from build123d import *

# Parameters (mm, degrees)
CROQUIS1_W              = 70
CROQUIS1_H              = 70
CROQUIS1_R              = 25.5
SALIENTE_EXTRUIR1_DEPTH = 2
CROQUIS2_R              = 27.5
CROQUIS2_R_2            = 25.5
SALIENTE_EXTRUIR2_DEPTH = 3
CROQUIS3_W              = 70
CROQUIS3_H              = 17
CORTAR_EXTRUIR1_DEPTH   = 50.749371855


with BuildPart() as part:
    # Croquis1 → Saliente-Extruir1 (new body)
    with BuildSketch(Plane(origin=(0, 0, 0), x_dir=(1, 0, 0), z_dir=(0, 1, 0))):
        Rectangle(CROQUIS1_W, CROQUIS1_H)
        with Locations(Location((0, 0, 0), (0, 0, 270))):
            Circle(CROQUIS1_R, mode=Mode.SUBTRACT)
    extrude(amount=SALIENTE_EXTRUIR1_DEPTH)

    # Croquis2 → Saliente-Extruir2 (add)
    with BuildSketch(Plane(origin=(0, 2, 0), x_dir=(1, 0, 0), z_dir=(0, 1, 0))):
        with Locations(Location((0, 0, 0), (0, 0, 270))):
            Circle(CROQUIS2_R)
        with Locations(Location((0, 0, 0), (0, 0, 270))):
            Circle(CROQUIS2_R_2, mode=Mode.SUBTRACT)
    extrude(amount=SALIENTE_EXTRUIR2_DEPTH)

    # Croquis3 → Cortar-Extruir1 (cut, through all)
    with BuildSketch(Plane(origin=(0, 5, 0), x_dir=(1, 0, 0), z_dir=(0, 1, 0))):
        with Locations((0, -26.5)):
            Rectangle(CROQUIS3_W, CROQUIS3_H)
    extrude(amount=-CORTAR_EXTRUIR1_DEPTH, mode=Mode.SUBTRACT)


solid = part.part
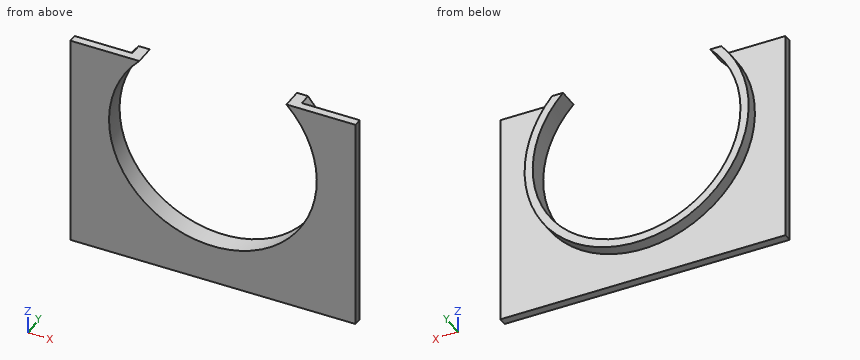
Design review of the part built by this model. Coordinates are the model's own, in mm. Give positions to 0.01 mm unless a question says otherwise; leave off trailing zeros. Order: outer loops, then holes, each group sorted by start corner. A loop starts at its lowest first (then second) coordinate and runs counter-clockwise, first axis right, second up. Notation, with made-up numbers: (16, 8.5) - (46, 8.5) arc R16 cw to (46, 34.5) - close; hole circle Ø1 at (-38, 85). An arc over 180 degrees is marked (long way). Use CSV: the item, a comma, the result in double quotes. Start each with the question number.
Q1. Take a section at A-A (z = 0). State the section outline as (x, y) points, and give its area (3 significant figures).
Q2. For line 1 (X direction, y = 1.8, z = 0); line 2 (X direction, y = 3.15, z = 0); line 3 (Y direction, x = 28.5, z = 5.5), list the stretches that pass through material, from the lowest coordinate up.
Q3. Take a section at B-B (y = 1.2). State the section outline as (x, z) points, and give its area (3 significant figures).
Q4. Take a section at D-D (x = 0). State the section outline as (y, z) points.
Q5. For P1, Ø1.5, axis at y = 4.5, z = -6, coming from the +X side, flat-tipped, find the tip position at first contact; note if it passes through.
Q6. Take a section at C-C (x = -20). State the section outline as (y, z) points, and give its area (3 significant figures).
Calculated:
1,outline,"(-35, 0) - (-25.5, 0) - (-25.5, 5) - (-27.5, 5) - (-27.5, 2) - (-35, 2) - close; (25.5, 0) - (35, 0) - (35, 2) - (27.5, 2) - (27.5, 5) - (25.5, 5) - close"
1,area,"50.0 mm²"
2,line 1,"x = -35 to -25.5, 25.5 to 35"
2,line 2,"x = -27.5 to -25.5, 25.5 to 27.5"
2,line 3,"y = 0 to 2"
3,outline,"(-35, -35) - (35, -35) - (35, 18) - (18.06, 18) arc R25.5 cw (long way) to (-18.06, 18) - (-35, 18) - close"
3,area,"1,850 mm²"
4,outline,"(0, -35) - (2, -35) - (2, -27.5) - (5, -27.5) - (5, -25.5) - (0, -25.5) - close"
5,P1,"stops at x = 26.99"
6,outline,"(0, -35) - (2, -35) - (2, -18.87) - (5, -18.87) - (5, -15.82) - (0, -15.82) - close; (0, 15.82) - (5, 15.82) - (5, 18) - (0, 18) - close"
6,area,"58.4 mm²"
